Here's how the part is built. I have some questions about the finished solid (model axes, mm). A direction names the side the tool comes from. Coordinates: 2 decimals unless noted, no trailing zeros. Write each loop counter-clockwise with the first axis right and the second up, starting at its lowest first coordinate (ties: lowest second). Pieces come first, ordered by that corner, then holes. Notation, with made-up numbers: M 1.25,-26 L 10.25,-26 A21 cw 10.25,-6 Z; hole C -2,4.5 d4. An arc over 180 degrees is marked long. Use a Markdown table: item, result.
```python
from build123d import *

# Parameters (mm, degrees)
SKETCH1_W           = 38.1
SKETCH1_H           = 25.4
BOSS_EXTRUDE1_DEPTH = 25.4
SKETCH4_R           = 0.635
CUT_EXTRUDE1_DEPTH  = 35.195796525
CUT_EXTRUDE2_DEPTH  = 1.5875
CUT_EXTRUDE3_DEPTH  = 3.175
FILLET1_R           = 3.302
FILLET2_R           = 0.8128
CHAMFER1_SIZE       = 0.635


with BuildPart() as part:
    # Sketch1 → Boss-Extrude1 (new body)
    with BuildSketch(Plane(origin=(0, 0, 0), x_dir=(1, 0, 0), z_dir=(0, 1, 0))):
        Rectangle(SKETCH1_W, SKETCH1_H)
    extrude(amount=BOSS_EXTRUDE1_DEPTH)

    # Sketch4 → Cut-Extrude1 (cut, through all)
    with BuildSketch(Plane(origin=(0, 25.4, 0), x_dir=(1, 0, 0), z_dir=(0, 1, 0))):
        with Locations(Location((-9.9568, -5.2959, 0), (0, 0, 270))):
            Circle(SKETCH4_R)
        with Locations(Location((-5.3594, -5.0419, 0), (0, 0, 270))):
            Circle(SKETCH4_R)
        with Locations(Location((-4.5974, 0.1143, 0), (0, 0, 270))):
            Circle(SKETCH4_R)
        with Locations(Location((-6.8326, 1.5113, 0), (0, 0, 270))):
            Circle(SKETCH4_R)
        with Locations(Location((-1.4478, 3.9751, 0), (0, 0, 270))):
            Circle(SKETCH4_R)
        with Locations(Location((-1.4224, 2.3749, 0), (0, 0, 270))):
            Circle(SKETCH4_R)
        with Locations(Location((5.4356, 0.8255, 0), (0, 0, 270))):
            Circle(SKETCH4_R)
        with Locations(Location((7.0612, 3.1877, 0), (0, 0, 270))):
            Circle(SKETCH4_R)
    extrude(amount=-CUT_EXTRUDE1_DEPTH, mode=Mode.SUBTRACT)

    # Sketch5 → Cut-Extrude2 (cut)
    with BuildSketch(Plane(origin=(0, 25.4, 0), x_dir=(1, 0, 0), z_dir=(0, 1, 0))):
        with BuildLine():
            Line((-15.164283352, 8.851416648), (-14.072566704, 7.7597))
            Line((-14.072566704, 7.7597), (14.100557504, 7.7597))
            Line((14.100557504, 7.7597), (15.192274152, 8.851416648))
            ThreePointArc((15.192274152, 8.851416648), (16.359707448, 8.851416648), (16.359707448, 7.683983352))
            Line((16.359707448, 7.683983352), (15.2679908, 6.592266704))
            Line((15.2679908, 6.592266704), (15.2679908, -6.580862104))
            Line((15.2679908, -6.580862104), (16.359707448, -7.672578752))
            ThreePointArc((16.359707448, -7.672578752), (16.359707448, -8.840012048), (15.192274152, -8.840012048))
            Line((15.192274152, -8.840012048), (14.100557504, -7.7482954))
            Line((14.100557504, -7.7482954), (-14.072566704, -7.7482954))
            Line((-14.072566704, -7.7482954), (-15.164283352, -8.840012048))
            ThreePointArc((-15.164283352, -8.840012048), (-16.331716648, -8.840012048), (-16.331716648, -7.672578752))
            Line((-16.331716648, -7.672578752), (-15.24, -6.580862104))
            Line((-15.24, -6.580862104), (-15.24, 6.592266704))
            Line((-15.24, 6.592266704), (-16.331716648, 7.683983352))
            ThreePointArc((-16.331716648, 7.683983352), (-16.331716648, 8.851416648), (-15.164283352, 8.851416648))
        make_face()
    extrude(amount=-CUT_EXTRUDE2_DEPTH, mode=Mode.SUBTRACT)

    # Sketch6 → Cut-Extrude3 (cut)
    with BuildSketch(Plane.XZ):
        Polygon((-19.05, -3.175), (-19.05, 3.175), (-16.51, 3.175), (-16.51, 10.16), (16.51, 10.16), (16.51, -10.16), (-16.51, -10.16), (-16.51, -3.175), align=None)
    extrude(amount=-CUT_EXTRUDE3_DEPTH, mode=Mode.SUBTRACT)

    # Fillet1
    fillet1_edges = [part.edges().sort_by_distance(p)[0] for p in [
        (-16.51, 1.5875, 10.16),
        (16.51, 1.5875, 10.16),
        (16.51, 1.5875, -10.16),
        (-16.51, 1.5875, -10.16),
    ]]
    fillet(fillet1_edges, radius=FILLET1_R)

    # Fillet2
    fillet2_edges = [part.edges().sort_by_distance(p)[0] for p in [
        (-16.51, 1.5875, 3.175),
        (-16.51, 1.5875, -3.175),
        (-19.05, 12.7, -12.7),
        (19.05, 12.7, -12.7),
        (19.05, 12.7, 12.7),
        (-19.05, 12.7, 12.7),
    ]]
    fillet(fillet2_edges, radius=FILLET2_R)

    # Chamfer1
    # the kernel refuses this chamfer: 0.635 mm, written as the material it takes off along each edge
    with BuildSketch(Plane(origin=(-5.3594, 3.175, 5.0419), x_dir=(0, 0, 1), z_dir=(-1, 0, 0))) as chamfer1_piece_1:
        Polygon((0.635 + CHAMFER1_SIZE, 0), (0.635, CHAMFER1_SIZE), (0.635, 0), align=None)
    revolve(axis=Axis((-5.3594, 3.175, 5.0419), (0, 1, 0)), mode=Mode.SUBTRACT)
    with BuildSketch(Plane(origin=(-6.8326, 3.175, -1.5113), x_dir=(0, 0, 1), z_dir=(-1, 0, 0))) as chamfer1_piece_2:
        Polygon((0.635 + CHAMFER1_SIZE, 0), (0.635, CHAMFER1_SIZE), (0.635, 0), align=None)
    revolve(axis=Axis((-6.8326, 3.175, -1.5113), (0, 1, 0)), mode=Mode.SUBTRACT)
    with BuildSketch(Plane(origin=(-1.4224, 3.175, -2.3749), x_dir=(0, 0, 1), z_dir=(-1, 0, 0))) as chamfer1_piece_3:
        Polygon((0.635 + CHAMFER1_SIZE, 0), (0.635, CHAMFER1_SIZE), (0.635, 0), align=None)
    revolve(axis=Axis((-1.4224, 3.175, -2.3749), (0, 1, 0)), mode=Mode.SUBTRACT)
    with BuildSketch(Plane(origin=(7.0612, 3.175, -3.1877), x_dir=(0, 0, 1), z_dir=(-1, 0, 0))) as chamfer1_piece_4:
        Polygon((0.635 + CHAMFER1_SIZE, 0), (0.635, CHAMFER1_SIZE), (0.635, 0), align=None)
    revolve(axis=Axis((7.0612, 3.175, -3.1877), (0, 1, 0)), mode=Mode.SUBTRACT)
    with BuildSketch(Plane(origin=(5.4356, 3.175, -0.8255), x_dir=(0, 0, 1), z_dir=(-1, 0, 0))) as chamfer1_piece_5:
        Polygon((0.635 + CHAMFER1_SIZE, 0), (0.635, CHAMFER1_SIZE), (0.635, 0), align=None)
    revolve(axis=Axis((5.4356, 3.175, -0.8255), (0, 1, 0)), mode=Mode.SUBTRACT)
    with BuildSketch(Plane(origin=(-1.4478, 3.175, -3.9751), x_dir=(0, 0, 1), z_dir=(-1, 0, 0))) as chamfer1_piece_6:
        Polygon((0.635 + CHAMFER1_SIZE, 0), (0.635, CHAMFER1_SIZE), (0.635, 0), align=None)
    revolve(axis=Axis((-1.4478, 3.175, -3.9751), (0, 1, 0)), mode=Mode.SUBTRACT)
    with BuildSketch(Plane(origin=(-4.5974, 3.175, -0.1143), x_dir=(0, 0, 1), z_dir=(-1, 0, 0))) as chamfer1_piece_7:
        Polygon((0.635 + CHAMFER1_SIZE, 0), (0.635, CHAMFER1_SIZE), (0.635, 0), align=None)
    revolve(axis=Axis((-4.5974, 3.175, -0.1143), (0, 1, 0)), mode=Mode.SUBTRACT)
    with BuildSketch(Plane(origin=(-9.9568, 3.175, 5.2959), x_dir=(0, 0, 1), z_dir=(-1, 0, 0))) as chamfer1_piece_8:
        Polygon((0.635 + CHAMFER1_SIZE, 0), (0.635, CHAMFER1_SIZE), (0.635, 0), align=None)
    revolve(axis=Axis((-9.9568, 3.175, 5.2959), (0, 1, 0)), mode=Mode.SUBTRACT)


solid = part.part
```
1. We'd pull the mould along Z, two halves only. Please class faces 1 (the face through (-1, 3.175, 0)), 2 (the face through (-1.5, 0, -10.4)): +Z half, -Z half, draft (parallel to the pull), parting line (faces both ways), or undercut.
Answers follow:
| item | result |
|---|---|
| face 1 | undercut |
| face 2 | draft |
2. Will these pins go through, and if not, where does the flat tip stop? pin 1 Ø1 at (x, z) = (-9.5, -4) entering from -Y (3 decimals); pin 2 Ø1 at (x, z) = (14, 4.5) entering from +Y; pin 3 Ø2 at (x, z) = (-6.83, -1.51) entering from -Y.
Answers follow:
| item | result |
|---|---|
| pin 1 | stops at y = 3.175 |
| pin 2 | stops at y = 23.81 |
| pin 3 | stops at y = 3.44 |
3. Which directions (+Z, -Z, +X, -X, +Y, -Y) give clear straight access to the entire face, cutting with the end or side of a thin tool? Please do faces 3 (the face through (16.51, 2, 0)), 4 (the face through (0, 25, 7.748)), 5 (the face through (-9.4, 14, 5.6)), 6 (the face through (-18, 2, -3.175)).
Answers follow:
| item | result |
|---|---|
| face 3 | -Y |
| face 4 | +Y |
| face 5 | +Y, -Y |
| face 6 | -X, -Y |
4. Suppose I cut it at A-A on x = 2.5. Write out the boundary of the cut face in (y, z) (1 decimal), and give its area (3 significant figures).
Answers follow:
| item | result |
|---|---|
| outline | M 0,-12.7 L 25.4,-12.7 L 25.4,-7.8 L 23.8,-7.8 L 23.8,7.7 L 25.4,7.7 L 25.4,12.7 L 0,12.7 L 0,10.2 L 3.2,10.2 L 3.2,-10.2 L 0,-10.2 Z |
| area | 556 mm2 |
5. I need wall thicknesses on probe 1 along Z at (x, y) = (-5, 1.5); probe 2 along X at (y, z) = (19.5, 5.5); probe 3 along X at (y, z) = (10, -0.5). Which ranges of each line are inside material? Lowest first, please.
Answers follow:
| item | result |
|---|---|
| probe 1 | z = -12.7 to -10.16, 10.16 to 12.7 |
| probe 2 | x = -19.05 to -10.56, -9.36 to -5.8, -4.92 to 19.05 |
| probe 3 | x = -19.05 to -5.1, -4.09 to 4.89, 5.98 to 19.05 |
